Can you work these out from the model? Positions are in its coordinate system, mm. A direction names the side the tool comes from. Give positions to 0.01 mm unless a question says otherwise; leave off trailing zeros. Write each loop counter-clockwise with the first axis right and the second up, starting at its lowest first coordinate (ties: lowest second). Pieces come first, ordered by that corner, then holes. Notation, with made-up numbers: (-21.5, 64.25) -> (-0.5, 64.25) arc R22 ccw to (-0.5, 88.25) -> close; hole circle Ø6 at (-9.75, 85.25). An arc over 180 degrees is marked (long way). Answer as CSV lines item,"result". Start each with the question number.
1. If we section it at A-A on x = 0: Write out the boundary of the cut face in (y, z), plus the area to 3 significant figures.
2. I need wall thicknesses on line 1 (Y direction, x = 0, z = 6.5); line 2 (Z direction, x = 9, y = -3); line 3 (X direction, y = -1.25, z = 7). Which ranges of each line are inside material? Lowest first, please. Write a range as [from, to].
3. If we section it at B-B on y = 0: Write out the boundary of the cut face in (x, z).
4. I'm going to push flat-ended pins straight in: P1, Ø1.5, axis at y = -2.5, z = 1.5, coming from the -X side; P2, Ø4.5, axis at x = 0, y = 0, coming from the -Z side; P3, Ø4, axis at x = 21, y = -3, coming from the +Z side. Where does each tip first touch, or does it pass through?
5. If we section it at D-D on z = 0.75: Write out the boundary of the cut face in (x, y), plus the area to 3 significant figures.
6. On a 3-axis mill with a long thin cutter (end or side, diameter ignored), from which of +Z, -Z, +X, -X, +Y, -Y can I reach the whole of each face in a straight line? I mean faces 1 (the face through (0, -3, 7.5)), 2 (the face through (-2.8, 0.1, 6.5)). Say none if no direction works.
7. If we mould it in two halves opening along Y, with no side actions, what happens to faces 3 (the face through (18, 0, 0)), 4 (the face through (20.71, 5.706, 0.986)), 5 (the face through (0, 0, 5.5))? For each: pulls with the +Y half, pulls with the -Y half, needs draft (parallel to the pull), parting line crosses it, or undercut.
8. If we section it at C-C on z = 5: Write out the boundary of the cut face in (x, y), plus the area to 3 significant figures.
```python
from build123d import *

# Parameters (mm, degrees)
SKETCH002_R      = 4.5
EXTRUDE002_DEPTH = 2
SKETCH_R         = 7
EXTRUDE001_DEPTH = 7.5
EXTRUDE_DEPTH    = 2
SKETCH003_R      = 2.8
POCKET_DEPTH     = 2


with BuildPart() as extrudehead:
    # Sketch002 → Extrude002 (new body)
    with BuildSketch(Plane.XY):
        with Locations((40, 0)):
            Circle(SKETCH002_R)
    extrude(amount=EXTRUDE002_DEPTH)


with BuildPart() as extrudemount:
    # Sketch → Extrude001 (new body)
    with BuildSketch(Plane.XY):
        Circle(SKETCH_R)
    extrude(amount=EXTRUDE001_DEPTH)


with BuildPart() as body:
    # Sketch001 (on Sketch) → Extrude (new body)
    with BuildSketch(Plane.XY):
        Polygon((40, 4.5), (0, 7), (0, -7), (40, -4.5), align=None)
    extrude(amount=EXTRUDE_DEPTH)

    # Fusion: union ExtrudeMount
    add(extrudemount.part)

    # Fusion001: union ExtrudeHead
    add(extrudehead.part)

    # Sketch003 (on Face16 of Fusion001) → Pocket (cut)
    with BuildSketch(Plane.XY.offset(7.5)):
        Circle(SKETCH003_R)
    extrude(amount=-POCKET_DEPTH, mode=Mode.SUBTRACT)


solid = body.part
```
Computed values:
1,outline,"(-7, 0) -> (7, 0) -> (7, 7.5) -> (2.8, 7.5) -> (2.8, 5.5) -> (-2.8, 5.5) -> (-2.8, 7.5) -> (-7, 7.5) -> close"
1,area,"93.8 mm2"
2,line 1,"y = [-7, -2.8], [2.8, 7]"
2,line 2,"z = [0, 2]"
2,line 3,"x = [-6.89, -2.51], [2.51, 6.89]"
3,outline,"(-7, 0) -> (44.5, 0) -> (44.5, 2) -> (7, 2) -> (7, 7.5) -> (2.8, 7.5) -> (2.8, 5.5) -> (-2.8, 5.5) -> (-2.8, 7.5) -> (-7, 7.5) -> close"
4,P1,"stops at x = -6.78"
4,P2,"stops at z = 0"
4,P3,"stops at z = 2"
5,outline,"(0.87, -6.95) -> (40, -4.5) arc R4.5 ccw to (40, 4.5) -> (0.87, 6.95) arc R7 ccw (long way) to start"
5,area,"569 mm2"
6,face 1,"+Z, +X, -X, +Y, -Y"
6,face 2,"+Z"
7,face 3,"needs draft"
7,face 4,"pulls with the +Y half"
7,face 5,"undercut"
8,outline,"circle Ø14 at (0, 0)"
8,area,"154 mm2"
